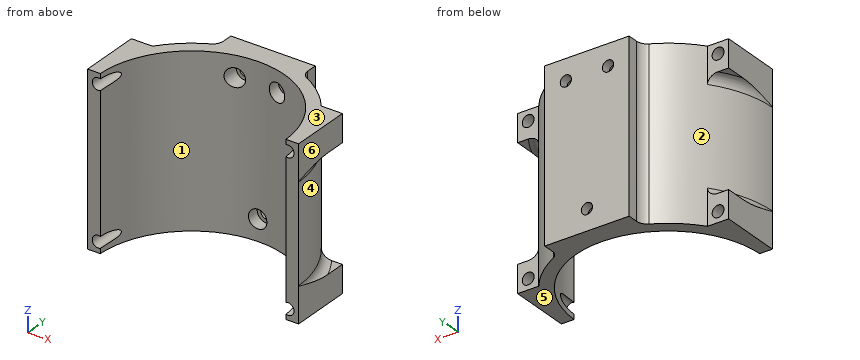
from build123d import *

# Parameters (mm, degrees)
BOSS_EXTRUDE1_DEPTH                          = 50.8
BOSS_EXTRUDE2_START                          = -16.51
BOSS_EXTRUDE2_DEPTH                          = 16.51
SKETCH4_W                                    = 127
SKETCH4_H                                    = 1.27
CUT_EXTRUDE1_DEPTH                           = 136.598893801
F_1_4_CLEARANCE_HOLE1_D                      = 7.14248
FILLET1_R                                    = 5.08
SKETCH7_W                                    = 50.8
SKETCH7_H                                    = 12.7
BOSS_EXTRUDE3_DEPTH                          = 101.6
FILLET2_R                                    = 6.35
CBORE_START                                  = 52.832
CBORE_FOR_1_4_SOCKET_HEAD_CAP_SCREW1_OUT_R   = 5.55625
CBORE_FOR_1_4_SOCKET_HEAD_CAP_SCREW1_DEPTH   = 10.16
CBORE_START_2                                = 62.992
CBORE_FOR_1_4_SOCKET_HEAD_CAP_SCREW1_2_O_R   = 3.3782
CBORE_FOR_1_4_SOCKET_HEAD_CAP_SCREW1_2_DEPTH = 5.588


# Read off the part's stored shape, not the designer's step: CBORE for 1/4 Socket Head Cap Screw1
with BuildPart() as part:
    # Sketch1 → Boss-Extrude1 (new, symmetric)
    with BuildSketch(Plane.XY):
        with BuildLine():
            Line((55.88, 0), (63.5, 0))
            ThreePointArc((63.5, 0), (0, 63.5), (-63.5, 0))
            Line((-63.5, 0), (-55.88, 0))
            ThreePointArc((-55.88, 0), (0, 55.88), (55.88, 0))
        make_face()
    extrude(amount=BOSS_EXTRUDE1_DEPTH, both=True)

    # Sketch2 → Boss-Extrude2 (add)
    with BuildSketch(Plane(origin=(0, 0, -50.8), x_dir=(-1, 0, 0), z_dir=(0, 0, -1)).offset(BOSS_EXTRUDE2_START)):
        with BuildLine():
            Line((-63.5, 38.1), (-63.5, 0))
            ThreePointArc((-63.5, 0), (-60.241389426, 20.080463142), (-50.8, 38.1))
            Line((-50.8, 38.1), (-63.5, 38.1))
        make_face()
        with BuildLine():
            Line((63.5, 38.1), (50.8, 38.1))
            ThreePointArc((50.8, 38.1), (60.241389426, 20.080463142), (63.5, 0))
            Line((63.5, 0), (63.5, 38.1))
        make_face()
    boss_extrude2 = extrude(amount=BOSS_EXTRUDE2_DEPTH)

    # Mirror1: Boss-Extrude2 across plane
    add(boss_extrude2.mirror(Plane.XY))

    # Sketch4 → Cut-Extrude1 (cut, through all)
    with BuildSketch(Plane.XY.offset(50.8)):
        with Locations((0, 0.635)):
            Rectangle(SKETCH4_W, SKETCH4_H)
    extrude(amount=-CUT_EXTRUDE1_DEPTH, mode=Mode.SUBTRACT)

    # 1/4 Clearance Hole1 (through all)
    with Locations(Plane(origin=(-57.15, 38.1, -44.45), x_dir=(0, 0, 1), z_dir=(0, 1, 0))):
        with Locations((0, 0), (0, 114.3), (88.9, 0), (88.9, 114.3)):
            Hole(F_1_4_CLEARANCE_HOLE1_D / 2)

    # Fillet1
    fillet1_edges = [part.edges().sort_by_distance(p)[0] for p in [
        (60.037562307, 20.681903014, 34.29),
        (-60.037562307, 20.681903014, 34.29),
        (-60.037562307, 20.681903014, -34.29),
        (60.037562307, 20.681903014, -34.29),
    ]]
    fillet(fillet1_edges, radius=FILLET1_R)

    # Sketch7 → Boss-Extrude3 (add)
    with BuildSketch(Plane(origin=(0, 0, -50.8), x_dir=(-1, 0, 0), z_dir=(0, 0, -1))):
        with Locations((0, 62.23)):
            Rectangle(SKETCH7_W, SKETCH7_H)
    extrude(amount=-BOSS_EXTRUDE3_DEPTH)

    # Fillet2
    fillet2_edges = [part.edges().sort_by_distance(p)[0] for p in [
        (-25.4, 58.198711326, 0),
        (25.4, 58.198711326, 0),
    ]]
    fillet(fillet2_edges, radius=FILLET2_R)

    # CBORE for 1/4 Socket Head Cap Screw1 out → CBORE for 1/4 Socket Head Cap Screw1 (cut)
    with BuildSketch(Plane(origin=(0, 0, 0), x_dir=(1, 0, 0), z_dir=(0, 1, 0)).offset(CBORE_START)):
        with Locations((-12.7, -38.1)):
            Circle(CBORE_FOR_1_4_SOCKET_HEAD_CAP_SCREW1_OUT_R)
        with Locations((12.7, -38.1)):
            Circle(CBORE_FOR_1_4_SOCKET_HEAD_CAP_SCREW1_OUT_R)
        with Locations((0, 38.1)):
            Circle(CBORE_FOR_1_4_SOCKET_HEAD_CAP_SCREW1_OUT_R)
    extrude(amount=CBORE_FOR_1_4_SOCKET_HEAD_CAP_SCREW1_DEPTH, mode=Mode.SUBTRACT)

    # CBORE for 1_4 Socket Head Cap Screw1 2 o → CBORE for 1_4 Socket Head Cap Screw1 2 (cut)
    with BuildSketch(Plane(origin=(0, 0, 0), x_dir=(1, 0, 0), z_dir=(0, 1, 0)).offset(CBORE_START_2)):
        with Locations((-12.7, -38.1)):
            Circle(CBORE_FOR_1_4_SOCKET_HEAD_CAP_SCREW1_2_O_R)
        with Locations((12.7, -38.1)):
            Circle(CBORE_FOR_1_4_SOCKET_HEAD_CAP_SCREW1_2_O_R)
        with Locations((0, 38.1)):
            Circle(CBORE_FOR_1_4_SOCKET_HEAD_CAP_SCREW1_2_O_R)
    extrude(amount=CBORE_FOR_1_4_SOCKET_HEAD_CAP_SCREW1_2_DEPTH, mode=Mode.SUBTRACT)


solid = part.part
Read the model definition and answer for the solid it produces. Units are mm, in the model's axes. Face numbers are marked on the shaded views. A direction names the side the tool comes from. Give positions to 0.01 mm unless a question says otherwise; leave off trailing zeros. Loops run counter-clockwise (first coordinate to the right, second up) from the corner with the lowest first, then second, coordinate; pieces in that order, holes last. Notation, with made-up numbers: (64.25, 23.5) - (97.25, 23.5) arc R16 ccw to (97.25, 41.5) - close; hole circle Ø4 at (63.25, 77.25). An arc over 180 degrees is marked (long way). Answer as CSV lines item,"result". Start each with the question number.
1) Straight lines are drawn through the part: L1, parallel to Z at x = -57, y = 27; L2, parallel to X at y = 57.5, z = 38.1; L3, parallel to Z at x = 0, y = 60. For each, find the intervals that lie inside material, in ascending order. Write a range as from..to.
2) Find section D-D (x = -35). Write down the section's boundary in (y, z), then the cut area to 3 significant figures.
3) Determine the mould class of the marked faces 3, 4, 5 and 6 for opening direction Z: released by +Z, released by -Z, zero draft, split by the parting line, or undercut.
4) Which of the six approach directions +Z, -Z, +X, -X, +Y, -Y give full straight-line access (tool end or side, diameter ignored) to the marked faces 1 and 2?
5) Find section A-A (z = -38.1). Write down the section's boundary in (x, y).
6) Each of these flat-tipped pins is pushed along its axis until it touches: pin 1 Ø5 at (x, z) = (12.5, 31.5) entering from -Y; pin 2 Ø11.5 at (x, z) = (-57.15, -44.45) entering from +Y; pin 3 Ø10 at (x, z) = (55.5, -35.5) entering from +Y. Where does it stop, or does it pass through?
7) Find section C-C (y = 30). State how many separate pieces and enclosed holes the cut face has, then the cut area to 3 significant figures.
Findings below:
1,L1,"-50.8..-48.02, -40.88..40.88, 48.02..50.8"
1,L2,"-27.5..-18.26, -7.14..7.14, 18.26..27.5"
1,L3,"-50.8..-43.66, -32.54..50.8"
2,outline,"(43.56, -50.8) - (52.98, -50.8) - (52.98, 50.8) - (43.56, 50.8) - close"
2,area,"957 mm^2"
3,face 3,"released by +Z"
3,face 4,"undercut"
3,face 5,"released by -Z"
3,face 6,"zero draft"
4,face 1,"+Z, -Z, -Y"
4,face 2,"-X, +Y"
5,outline,"(-63.5, 1.27) - (-55.87, 1.27) arc R55.88 cw to (-5.56, 55.6) - (-5.56, 62.99) - (-3.38, 62.99) - (-3.38, 68.58) - (-25.4, 68.58) - (-25.4, 62.22) arc R6.35 cw to (-28.86, 56.56) arc R63.5 ccw to (-50.8, 38.1) - (-63.5, 38.1) - close; (3.38, 62.99) - (5.56, 62.99) - (5.56, 55.6) arc R55.88 cw to (55.87, 1.27) - (63.5, 1.27) - (63.5, 38.1) - (50.8, 38.1) arc R63.5 ccw to (28.86, 56.56) arc R6.35 cw to (25.4, 62.22) - (25.4, 68.58) - (3.38, 68.58) - close"
6,pin 1,"y = 53.83"
6,pin 2,"y = 38.1"
6,pin 3,"y = 38.5"
7,separate pieces,"2"
7,enclosed holes,"4"
7,area,"2,150 mm^2"
